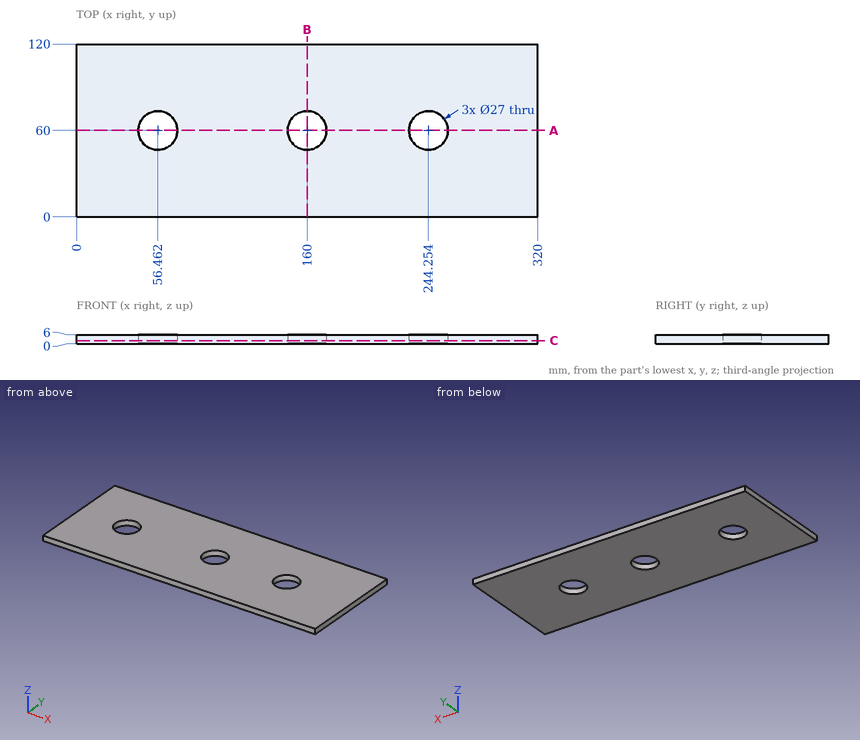
Design review of the part shown in the three views and the two pictorial views. Dimensions are in mm from the part's minimum x, y and z. Round coordinates to 2 decimals unless told otherwise and drop trailing zeros. Loops run counter-clockwise (first coordinate to the right, second up) from the corner with the lowest first, then second, coordinate; pieces in that order, holes last. Notation, with made-up numbers: (21.25, 39.25) -> (64.25, 39.25) arc R23 cw to (64.25, 70.25) -> close; hole circle Ø4 at (1, 55). An arc over 180 degrees is marked (long way). Use one line per item in the form item = value. Start each with the question number.
Q1. We need section A-A on y = 60. Give the boundary of the cut face in (x, z), then the cut area to 3 significant figures.
Q2. We need section C-C on z = 2. Give the boundary of the cut face in (x, y), then the cut area to 3 significant figures.
Q3. Wall thickness on line 1 along X through (y, z) = (60, 2.3); line 2 along Y through (x, z) = (160, 2.9); line 3 along X through (y, z) = (62, 0.75) (3 decimals): over which ranges is each line inside the solid? List them lowest first. Write a range as [from, to].
Q4. For pin 1 Ø16 at (x, y) = (56.46, 60) entering from +Z; pin 2 Ø8 at (x, y) = (128, 55.5) entering from -Z, all flat-tipped, find the tip position at first contact; note any pin that passes through.
Q5. We need section B-B on x = 160. Give the boundary of the cut face in (y, z), then the cut area to 3 significant figures.
Calculated:
q1.outline = (0, 0) -> (42.96, 0) -> (42.96, 6) -> (0, 6) -> close; (69.96, 0) -> (146.5, 0) -> (146.5, 6) -> (69.96, 6) -> close; (173.5, 0) -> (230.75, 0) -> (230.75, 6) -> (173.5, 6) -> close; (257.75, 0) -> (320, 0) -> (320, 6) -> (257.75, 6) -> close
q1.area = 1,430 mm²
q2.outline = (0, 0) -> (320, 0) -> (320, 120) -> (0, 120) -> close; hole circle Ø27 at (56.46, 60); hole circle Ø27 at (160, 60); hole circle Ø27 at (244.25, 60)
q2.area = 36,700 mm²
q3.line_1 = [0, 42.96], [69.96, 146.5], [173.5, 230.75], [257.75, 320]
q3.line_2 = [0, 46.5], [73.5, 120]
q3.line_3 = [0, 43.111], [69.813, 146.649], [173.351, 230.903], [257.605, 320]
q4.pin_1 = through
q4.pin_2 = 0
q5.outline = (0, 0) -> (46.5, 0) -> (46.5, 6) -> (0, 6) -> close; (73.5, 0) -> (120, 0) -> (120, 6) -> (73.5, 6) -> close
q5.area = 558 mm²
